The listing builds one solid part. Answer for the finished solid, in the listing's coordinates (mm). A direction names the side the tool comes from. Give positions to 0.01 mm unless a question says otherwise; leave off trailing zeros. Write each loop counter-clockwise with the first axis right and the second up, starting at its lowest first coordinate (ties: lowest second). Pieces come first, ordered by that corner, then holes. Notation, with made-up numbers: M -7,-13 L 30,-13 A28 cw 30,17 Z; hole C 22.5,6.25 d2. An arc over 180 degrees is marked long. Return JSON: item names as keys, results as strings.
Autodesk Fusion 360 part; units mm, degrees
sketch "Sketch1" plane through (0, 0, 0) normal (0, 0, 1) x (1, 0, 0)
  circle A0 centre (0, 0) radius 5.25
  line L0 (0, 0) -> (20, 0)
  circle A1 centre (20, 0) radius 5.25
  line L1 (0, 0) -> (-15, 0)
  line L2 (-15, 0) -> (-15, 15)
  line L3 (-15, 0) -> (-15, -15)
  line L4 (-15, -15) -> (55, -15)
  line L5 (-15, 15) -> (55, 15)
  line L6 (55, 15) -> (55, -15)
  circle A2 centre (-10, 0) radius 2.5
  dimension "d1" = 10.5
  dimension "d2" = 20
  dimension "d3" = 10.5
  dimension "d4" = 15
  dimension "d5" = 15
  dimension "d6" = 15
  dimension "d7" = 70
  dimension "d8" = 5
extrude "Extrude1" add sketch "Sketch1" along normal blind 8.5
sketch "Sketch2" plane through (0, 0, 8.5) normal (0, 0, 1) x (1, 0, 0)
  circle A0 centre (0, 0) radius 5.25
  circle A1 centre (-10, 0) radius 2.5
  circle A2 centre (20, 0) radius 5.25
  line L0 (-15, 15) -> (-15, -15)
  line L1 (-15, -15) -> (55, -15)
  line L2 (55, -15) -> (55, 15)
  line L3 (55, 15) -> (-15, 15)
  line L4 (-10, 10) -> (55, 10)
  line L5 (55, 10) -> (55, -10)
  line L6 (55, -10) -> (-10, -10)
  line L7 (-10, -10) -> (-10, 10)
  dimension "d11" = 20
  dimension "d12" = 65
extrude "Extrude2" add sketch "Sketch2" along normal blind 10 contours A1 L0 L1 L2 L3 L4 L6 L7
sketch "Sketch3" plane through (0, 0, 0) normal (0, 0, -1) x (-1, 0, 0)
  circle A0 centre (0, 0) radius 5.25
  circle A1 centre (10, 0) radius 2.5
  circle A2 centre (-20, 0) radius 5.25
  line L0 (15, -15) -> (15, 15)
  line L1 (15, 15) -> (-55, 15)
  line L2 (-55, 15) -> (-55, -15)
  line L3 (-55, -15) -> (15, -15)
  circle A3 centre (-20, 0) radius 7.25
  circle A4 centre (0, 0) radius 7.25
  dimension "d15" = 14.5
  dimension "d16" = 14.5
extrude "Extrude3" add sketch "Sketch3" along normal blind 2 contours L0 L1 L2 L3
chamfer "Chamfer1" distance 1 angle 45 16 edges at (20, 15, -2) (-15, 15, 8.25) (-15, 0, -2) (-15, -15, 8.25) (20, -15, -2) (55, 0, -2) (20, -15, 18.5) (-15, 0, 18.5) (20, 15, 18.5) (55, 15, 8.25) (55, -15, 8.25) (55, -12.5, 18.5) (55, 12.5, 18.5) (55, -10, 13.5) (55, 0, 8.5) (55, 10, 13.5)
chamfer "Chamfer2" distance 0.4 angle 45 5 edges at (22, -10, 18.5) (-10, -6.25, 18.5) (-12.5, 0, 18.5) (-10, 6.25, 18.5) (22, 10, 18.5)
Item 1: A cutting plane is placed at A-A, the plane z = 6.5. Write down the section's boundary in (x, y).
Geometry results:
{"outline": "M -15,-14 L -14,-15 L 54,-15 L 55,-14 L 55,14 L 54,15 L -14,15 L -15,14 Z; hole C -10,0 d5; hole C 0,0 d10.5; hole C 20,0 d10.5"}
Item 2: Which of the six approach directions +Z, -Z, +X, -X, +Y, -Y give full straight-line access (tool end or side, diameter ignored) to faces 1 (the flat face through (-10, -6, 13)), 2 (the flat face through (4, 4, 0)), 3 (the flat face through (28, 0, -2))?
Geometry results:
{"face 1": "+Z, +X", "face 2": "-Z", "face 3": "-Z, +X, -X, +Y, -Y"}
Item 3: Find the intervals of material crossed by line 1 (Y direction, x = 40.5, z = 10.5); line 2 (Y direction, x = 20, z = 4); line 3 (X direction, y = -2.25, z = 4.25), in increasing order.
Geometry results:
{"line 1": "y = -15 to -10, 10 to 15", "line 2": "y = -15 to -5.25, 5.25 to 15", "line 3": "x = -15 to -11.09, -8.91 to -4.74, 4.74 to 15.26, 24.74 to 55"}
Item 4: A cutting plane is placed at C-C, the plane x = 0. Write down the section's boundary in (y, z), plus the area to 3 significant figures.
Geometry results:
{"outline": "M -15,-1 L -14,-2 L -7.25,-2 L -7.25,0 L -5.25,0 L -5.25,8.5 L -10,8.5 L -10,18.1 L -10.4,18.5 L -14,18.5 L -15,17.5 Z; M 5.25,0 L 7.25,0 L 7.25,-2 L 14,-2 L 15,-1 L 15,17.5 L 14,18.5 L 10.4,18.5 L 10,18.1 L 10,8.5 L 5.25,8.5 Z", "area": "295 mm2"}
Item 5: Given pin 1 Ø4.5 at (x, y) = (-1, -1) entering from -Z; pin 2 Ø13 at (x, y) = (20, 0) entering from +Z; pin 3 Ø2 at (y, z) = (-6.5, 14) entering from +X, each flat-ended and moving along its own axis, determine where each tip first touches the part or whether it passes through.
Geometry results:
{"pin 1": "passes through", "pin 2": "stops at z = 8.5", "pin 3": "stops at x = -10"}
Item 6: Determine the mould class of faces 4 (the flat face through (24, 4, 0)), 5 (the flat face through (20, -15, 8)), 6 (the flat face through (-15, 0, 8)), 7 (the flat face through (20, 15, 8)) for opening direction Y: +Y half, -Y half, draft (parallel to the pull), parting line (faces both ways), or undercut.
Geometry results:
{"face 4": "undercut", "face 5": "-Y half", "face 6": "draft", "face 7": "+Y half"}
Item 7: A cutting plane is placed at D-D, the plane y = -8.75. Write down the section's boundary in (x, z).
Geometry results:
{"outline": "M -15,-1 L -14,-2 L 54,-2 L 55,-1 L 55,7.5 L 54,8.5 L -10,8.5 L -10,18.1 L -10.4,18.5 L -14,18.5 L -15,17.5 Z"}
Item 8: A cutting plane is placed at B-B, the plane y = 0. Count the separate pieces of the cut face and the enclosed holes in it, plus the area to 3 significant figures.
Geometry results:
{"separate pieces": "4", "enclosed holes": "0", "area": "469 mm2"}
